Part print with two shaded views. Sizes in mm from the minimum x, y, z corner. Give positions to 0.01 mm unless a question says otherwise; leave off trailing zeros. Order: outer loops, then holes, each group sorted by start corner. A loop starts at its lowest first (then second) coordinate and runs counter-clockwise, first axis right, second up. Notation, with made-up numbers: M 44,50 L 82,50 A10 ccw 82,54 Z; hole C 44,39.25 d8. An arc over 180 degrees is marked long. Return JSON: item names as keys, results as strings.
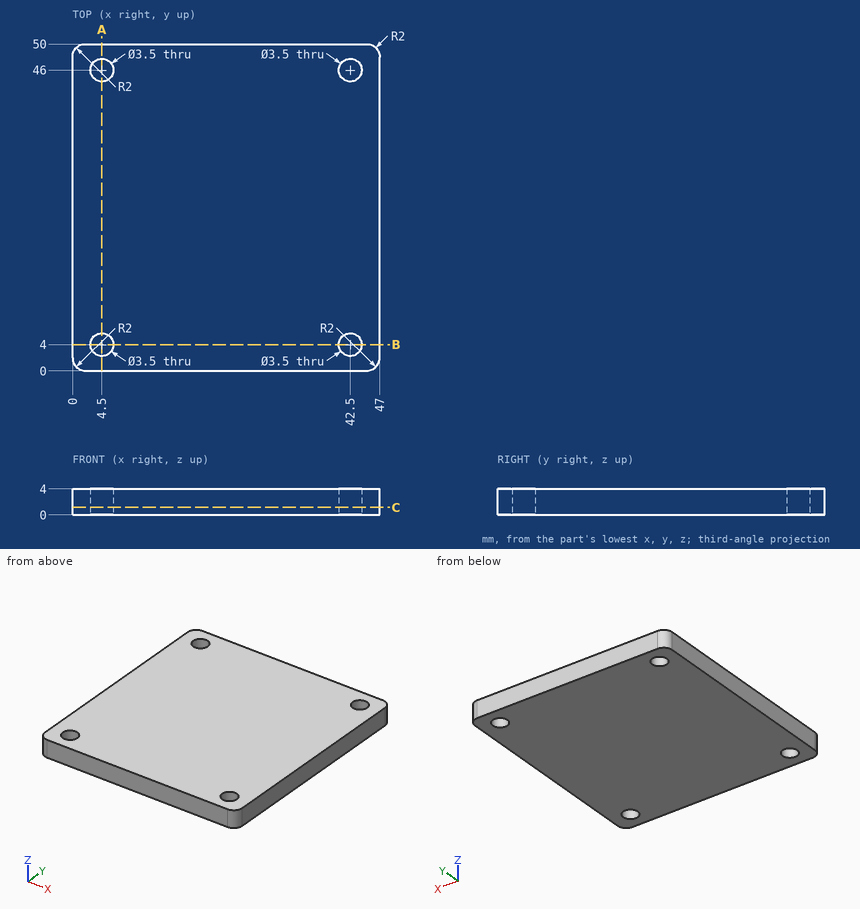
Q1. Pin check, flat tip, straight feed: pin 1 (1 mm diameter, centred on y = 23.5, z = 3, fed in from -X). Stop position of the tip, or through.
Established:
{"pin 1": "stops at x = 0"}
Q2. Band-saw the part on B-B (y = 4). Give the cut face in (x, z).
Established:
{"outline": "M 0,0 L 2.75,0 L 2.75,4 L 0,4 Z; M 6.25,0 L 40.75,0 L 40.75,4 L 6.25,4 Z; M 44.25,0 L 47,0 L 47,4 L 44.25,4 Z"}
Q3. Band-saw the part on A-A (x = 4.5). Give the cut face in (y, z).
Established:
{"outline": "M 0,0 L 2.25,0 L 2.25,4 L 0,4 Z; M 5.75,0 L 44.25,0 L 44.25,4 L 5.75,4 Z; M 47.75,0 L 50,0 L 50,4 L 47.75,4 Z"}
Q4. Band-saw the part on C-C (z = 1.15). Give the cut face in (x, y), then the cut area to 3 significant figures.
Established:
{"outline": "M 0,2 A2 ccw 2,0 L 45,0 A2 ccw 47,2 L 47,48 A2 ccw 45,50 L 2,50 A2 ccw 0,48 Z; hole C 4.5,4 d3.5; hole C 4.5,46 d3.5; hole C 42.5,4 d3.5; hole C 42.5,46 d3.5", "area": "2,310 mm²"}
Q5. Probe line 1 along Y through (x, z) = (4.5, 1.45); line 2 along X through (y, z) = (3, 1.8); line 3 along X through (y, z) = (44.5, 1.2). List the from-to ranges inside material, lowest first.
Established:
{"line 1": "y = 0 to 2.25, 5.75 to 44.25, 47.75 to 50", "line 2": "x = 0 to 3.06, 5.94 to 41.06, 43.94 to 47", "line 3": "x = 0 to 3.6, 5.4 to 41.6, 43.4 to 47"}
